Build history of the part. All positions in model axes, mm. A direction names the side the tool comes from. Give positions to 0.01 mm unless a question says otherwise; leave off trailing zeros. Loops run counter-clockwise (first coordinate to the right, second up) from the corner with the lowest first, then second, coordinate; pieces in that order, holes last. Notation, with made-up numbers: (82.5, 17.5) - (125.5, 17.5) arc R24 cw to (125.5, 33.5) - close; hole circle Ø5 at (63.5, -28.75). An arc over 180 degrees is marked (long way). Return JSON: item names as keys, results as strings. Group by question number.
1) Slice it at C-C (x = 13.5). List the corners of the cut face in (y, z), and give its area (3 significant figures).
2) Drill centre lines: probe 1 along Z at (x, y) = (20.5, -17); probe 2 along Z at (x, y) = (8.5, -13.25); probe 3 along X at (y, z) = (-10.75, 8.5). Where is each one in solid material? Low to high. Write a range as from..to.
3) Mould opens along X. For faces 1 (the face through (47, -9, 6)), 2 (the face through (3.955, -9.126, 4.646)), 3 (the face through (28, -18, 9)) say: released by +X, released by -X, zero draft, split by the parting line, or undercut.
4) Drop flat-ended pins along their axis: pin 1 (4 mm diameter, centred on x = 6, y = -11.5, fed in from +Z); pin 2 (9 mm diameter, centred on x = 24.5, y = -10, fed in from -Z); pin 3 (4 mm diameter, centred on y = -7, z = 10.5, fed in from -X). Give the stop position or say it passes through.
5) Slice it at D-D (z = 8.75). List the corners of the cut face in (x, y), and give its area (3 significant figures).
6) 3-axis set-ups, long thin cutter, end or side, ignore diameter. For faces 4 (the face through (32, -9, 12.5)), 5 (the face through (17, -9, 10)), 6 (the face through (43.146, -9.126, 4.545)): which of +Z, -Z, +X, -X, +Y, -Y reach the whole face in a straight line?
7) Slice it at A-A (z = 5.25). List the corners of the cut face in (x, y), and give its area (3 significant figures).
8) Slice it at B-B (y = -7.75). List the corners of the cut face in (x, z).
```python
from build123d import *

# Parameters (mm, degrees)
F0_W     = 47
F0_H     = 7.5
F1_DEPTH = 18
F2_W     = 30
F2_H     = 6.5
F3_DEPTH = 25
F4_R     = 6.5
F5_DEPTH = 25
F6_R     = 6.5
F7_DEPTH = 25
F8_W     = 30
F8_H     = 18
F9_DEPTH = 5


with BuildPart() as f1:
    # F0 (on Front) → F1 (new body)
    with BuildSketch(Plane.XZ):
        with Locations((23.5, 3.75)):
            Rectangle(F0_W, F0_H)
    extrude(amount=F1_DEPTH)

    # F2 (on face) → F3 (cut)
    with BuildSketch(Plane.XZ.offset(18)):
        with Locations((23.5, 3.25)):
            Rectangle(F2_W, F2_H)
    extrude(amount=-F3_DEPTH, mode=Mode.SUBTRACT)

    # F4 (on face) → F5 (cut)
    with BuildSketch(Plane.XZ.offset(18)):
        with Locations((8.5, 0)):
            Circle(F4_R)
    extrude(amount=-F5_DEPTH, mode=Mode.SUBTRACT)

    # F6 (on face) → F7 (cut)
    with BuildSketch(Plane.XZ.offset(18)):
        with Locations((38.5, 0)):
            Circle(F6_R)
    extrude(amount=-F7_DEPTH, mode=Mode.SUBTRACT)

    # F8 (on face) → F9 (join)
    with BuildSketch(Plane.XY.offset(7.5)):
        with Locations((32, -9)):
            Rectangle(F8_W, F8_H)
    extrude(amount=F9_DEPTH)


solid = f1.part
```
Results:
{
 "1": {"outline": "(-18, 6.5) - (0, 6.5) - (0, 7.5) - (-18, 7.5) - close", "area": "18.0 mm2"},
 "2": {"probe 1": "6.5..12.5", "probe 2": "6.5..7.5", "probe 3": "17..47"},
 "3": {"face 1": "released by +X", "face 2": "undercut", "face 3": "zero draft"},
 "4": {"pin 1": "z = 7.5", "pin 2": "z = 6.5", "pin 3": "x = 17"},
 "5": {"outline": "(17, -18) - (47, -18) - (47, 0) - (17, 0) - close", "area": "540 mm2"},
 "6": {"face 4": "+Z, +X, -X, +Y, -Y", "face 5": "+Z, -X, +Y, -Y", "face 6": "-Z, +Y, -Y"},
 "7": {"outline": "(0, -18) - (4.67, -18) - (4.67, 0) - (0, 0) - close; (42.33, -18) - (47, -18) - (47, 0) - (42.33, 0) - close", "area": "168 mm2"},
 "8": {"outline": "(0, 0) - (2, 0) arc R6.5 cw to (8.5, 6.5) - (38.5, 6.5) arc R6.5 cw to (45, 0) - (47, 0) - (47, 12.5) - (17, 12.5) - (17, 7.5) - (0, 7.5) - close"}
}
